from build123d import *

# Parameters (mm, degrees)
SKETCH1_W             = 76.2
SKETCH1_H             = 12.7
BOSS_EXTRUDE2_DEPTH   = 4.7625
F_4_CLEARANCE_HOLE1_D = 3.2639
CUT_EXTRUDE1_DEPTH    = 5.7625
CHAMFER1_SIZE         = 0.508


with BuildPart() as part:
    # Sketch1 → Boss-Extrude2 (new body)
    with BuildSketch(Plane(origin=(0, 0, 0), x_dir=(1, 0, 0), z_dir=(0, 1, 0))):
        with Locations((-31.75, 0)):
            Rectangle(SKETCH1_W, SKETCH1_H)
    extrude(amount=BOSS_EXTRUDE2_DEPTH)

    # #4 Clearance Hole1 (through all)
    with Locations(Plane(origin=(0, 4.7625, 0), x_dir=(1, 0, 0), z_dir=(0, 1, 0))):
        with Locations((-63.5, 0)):
            Hole(F_4_CLEARANCE_HOLE1_D / 2)

    # Sketch2 → Cut-Extrude1 (cut, through all)
    with BuildSketch(Plane(origin=(0, 4.7625, 0), x_dir=(1, 0, 0), z_dir=(0, 1, 0))):
        with BuildLine():
            ThreePointArc((3.1623, 0), (2.236083774, 2.236083774), (0, 3.1623))
            Line((0, 3.1623), (0, -3.1623))
            ThreePointArc((0, -3.1623), (2.236083774, -2.236083774), (3.1623, 0))
        make_face()
        with BuildLine():
            Line((0, -3.1623), (0, 3.1623))
            ThreePointArc((0, 3.1623), (-3.1623, 0), (0, -3.1623))
        make_face()
    extrude(amount=-CUT_EXTRUDE1_DEPTH, mode=Mode.SUBTRACT)

    # Chamfer1
    chamfer1_edges = [part.edges().sort_by_distance(p)[0] for p in [
        (-69.85, 2.38125, 6.35),
        (-69.85, 2.38125, -6.35),
        (6.35, 2.38125, -6.35),
        (6.35, 2.38125, 6.35),
        (6.35, 4.7625, 0),
        (-69.85, 4.7625, 0),
        (-69.85, 0, 0),
        (6.35, 0, 0),
    ]]
    chamfer(chamfer1_edges, length=CHAMFER1_SIZE)


solid = part.part
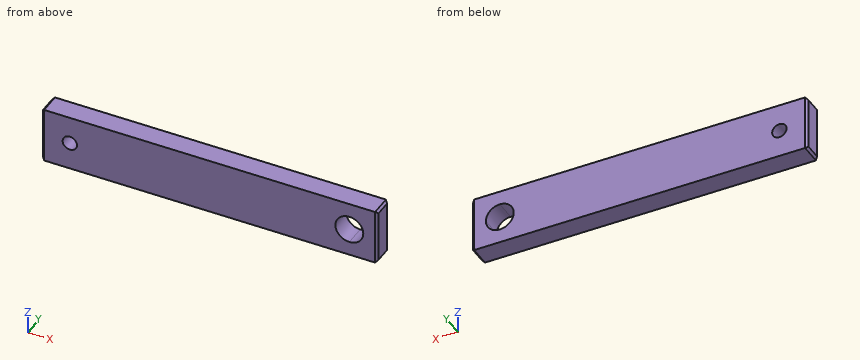
Input: part model. Units: mm. Frame: model coordinates. Coordinates: 2 decimals unless noted, no trailing zeros. Loops run counter-clockwise (first coordinate to the right, second up) from the corner with the lowest first, then second, coordinate; pieces in that order, holes last. Notation, with made-up numbers: (53, 30.25) - (109, 30.25) arc R12 ccw to (109, 44.25) - close; hole circle Ø8 at (-3.5, 44.25). An arc over 180 degrees is marked (long way). Answer in a Markdown table with one row per item. Add a question column.
Item 1: Contact query for a flat-ended pin moving along its axis: P1, Ø2, axis at x = -63.5, z = 0, coming from the -Y side. Output: stop coordinate, or through.
Item 2: Section query A-A on x = -63.5. Return the cut outline in (y, z).
Item 3: Section query B-B on y = 1.4. Return the cut outline in (x, z).
Item 4: Line query: line 1 along Z through (x, y) = (-63.5, 2.1); line 2 along Z through (x, y) = (2, 2); line 3 along X through (y, z) = (2.4, -2). Output: solid intervals per line, ascending. Write a range as [from, to].
Recorded:
| question | item | result |
|---|---|---|
| 1 | P1 | through |
| 2 | outline | (0, -6.35) - (4.76, -6.35) - (4.76, -1.63) - (0, -1.63) - close; (0, 1.63) - (4.76, 1.63) - (4.76, 6.35) - (0, 6.35) - close |
| 3 | outline | (-69.85, -5.84) - (-69.34, -6.35) - (5.84, -6.35) - (6.35, -5.84) - (6.35, 5.84) - (5.84, 6.35) - (-69.34, 6.35) - (-69.85, 5.84) - close; hole circle Ø3.26 at (-63.5, 0); hole circle Ø6.32 at (0, 0) |
| 4 | line 1 | [-6.35, -1.63], [1.63, 6.35] |
| 4 | line 2 | [-6.35, -2.45], [2.45, 6.35] |
| 4 | line 3 | [-69.85, -2.45], [2.45, 6.35] |
